from build123d import *

# Parameters (mm, degrees)
ESTRUSIONE_ESTRUSIONE1_DEPTH = 10
TAGLIO_ESTRUSIONE6_DEPTH     = 3.5
SCHIZZO3_R                   = 1.75
TAGLIO_ESTRUSIONE7_DEPTH     = 21.645708387
ESTRUSIONE_ESTRUSIONE2_DEPTH = 3
SCHIZZO5_R                   = 2
TAGLIO_ESTRUSIONE8_DEPTH     = 1.5
SMUSSO2_SIZE                 = 0.5
TAGLIO_ESTRUSIONE9_DEPTH     = 3.5


with BuildPart() as part:
    # Schizzo1 → Estrusione-Estrusione1 (new, symmetric)
    with BuildSketch(Plane.XY):
        Polygon((11, -1), (11, 0), (-11, 0), (-11, -1), (-15.041451884, -8), (-15.041451884, -10), (15.041451884, -10), (15.041451884, -8), align=None)
    extrude(amount=ESTRUSIONE_ESTRUSIONE1_DEPTH, both=True)

    # Schizzo2 → Taglio-Estrusione6 (cut, symmetric)
    with BuildSketch(Plane(origin=(0, 0, 0), x_dir=(0, 0, -1), z_dir=(1, 0, 0))):
        with BuildLine():
            Line((-10, 0), (-9.740175425, 0))
            ThreePointArc((-9.740175425, 0), (-9.641268354, -0.037228588), (-9.591456891, -0.130434783))
            ThreePointArc((-9.591456891, -0.130434783), (-9.557611714, -0.288062154), (-9.498876404, -0.438202247))
            ThreePointArc((-9.498876404, -0.438202247), (-9, -0.75), (-8.501123596, -0.438202247))
            ThreePointArc((-8.501123596, -0.438202247), (-8.442388286, -0.288062154), (-8.408543109, -0.130434783))
            ThreePointArc((-8.408543109, -0.130434783), (-8.358731646, -0.037228588), (-8.259824575, 0))
            Line((-8.259824575, 0), (-8, 0))
            Line((-8, 0), (-7.740175425, 0))
            ThreePointArc((-7.740175425, 0), (-7.641268354, -0.037228588), (-7.591456891, -0.130434783))
            ThreePointArc((-7.591456891, -0.130434783), (-7.557611714, -0.288062154), (-7.498876404, -0.438202247))
            ThreePointArc((-7.498876404, -0.438202247), (-7, -0.75), (-6.501123596, -0.438202247))
            ThreePointArc((-6.501123596, -0.438202247), (-6.442388286, -0.288062154), (-6.408543109, -0.130434783))
            ThreePointArc((-6.408543109, -0.130434783), (-6.358731646, -0.037228588), (-6.259824575, 0))
            Line((-6.259824575, 0), (-6, 0))
            Line((-6, 0), (-5.740175425, 0))
            ThreePointArc((-5.740175425, 0), (-5.641268354, -0.037228588), (-5.591456891, -0.130434783))
            ThreePointArc((-5.591456891, -0.130434783), (-5.557611714, -0.288062154), (-5.498876404, -0.438202247))
            ThreePointArc((-5.498876404, -0.438202247), (-5, -0.75), (-4.501123596, -0.438202247))
            ThreePointArc((-4.501123596, -0.438202247), (-4.442388286, -0.288062154), (-4.408543109, -0.130434783))
            ThreePointArc((-4.408543109, -0.130434783), (-4.358731646, -0.037228588), (-4.259824575, 0))
            Line((-4.259824575, 0), (-4, 0))
            Line((-4, 0), (-3.740175425, 0))
            ThreePointArc((-3.740175425, 0), (-3.641268354, -0.037228588), (-3.591456891, -0.130434783))
            ThreePointArc((-3.591456891, -0.130434783), (-3.557611714, -0.288062154), (-3.498876404, -0.438202247))
            ThreePointArc((-3.498876404, -0.438202247), (-3, -0.75), (-2.501123596, -0.438202247))
            ThreePointArc((-2.501123596, -0.438202247), (-2.442388286, -0.288062154), (-2.408543109, -0.130434783))
            ThreePointArc((-2.408543109, -0.130434783), (-2.358731646, -0.037228588), (-2.259824575, 0))
            Line((-2.259824575, 0), (-2, 0))
            Line((-2, 0), (-1.740175425, 0))
            ThreePointArc((-1.740175425, 0), (-1.641268354, -0.037228588), (-1.591456891, -0.130434783))
            ThreePointArc((-1.591456891, -0.130434783), (-1.557611714, -0.288062154), (-1.498876404, -0.438202247))
            ThreePointArc((-1.498876404, -0.438202247), (-1, -0.75), (-0.501123596, -0.438202247))
            ThreePointArc((-0.501123596, -0.438202247), (-0.442388286, -0.288062154), (-0.408543109, -0.130434783))
            ThreePointArc((-0.408543109, -0.130434783), (-0.358731646, -0.037228588), (-0.259824575, 0))
            Line((-0.259824575, 0), (0, 0))
            Line((0, 0), (0.259824575, 0))
            ThreePointArc((0.259824575, 0), (0.358731646, -0.037228588), (0.408543109, -0.130434783))
            ThreePointArc((0.408543109, -0.130434783), (0.442388286, -0.288062154), (0.501123596, -0.438202247))
            ThreePointArc((0.501123596, -0.438202247), (1, -0.75), (1.498876404, -0.438202247))
            ThreePointArc((1.498876404, -0.438202247), (1.557611714, -0.288062154), (1.591456891, -0.130434783))
            ThreePointArc((1.591456891, -0.130434783), (1.641268354, -0.037228588), (1.740175425, 0))
            Line((1.740175425, 0), (2, 0))
            Line((2, 0), (2.259824575, 0))
            ThreePointArc((2.259824575, 0), (2.358731646, -0.037228588), (2.408543109, -0.130434783))
            ThreePointArc((2.408543109, -0.130434783), (2.442388286, -0.288062154), (2.501123596, -0.438202247))
            ThreePointArc((2.501123596, -0.438202247), (3, -0.75), (3.498876404, -0.438202247))
            ThreePointArc((3.498876404, -0.438202247), (3.557611714, -0.288062154), (3.591456891, -0.130434783))
            ThreePointArc((3.591456891, -0.130434783), (3.641268354, -0.037228588), (3.740175425, 0))
            Line((3.740175425, 0), (4, 0))
            Line((4, 0), (4.259824575, 0))
            ThreePointArc((4.259824575, 0), (4.358731646, -0.037228588), (4.408543109, -0.130434783))
            ThreePointArc((4.408543109, -0.130434783), (4.442388286, -0.288062154), (4.501123596, -0.438202247))
            ThreePointArc((4.501123596, -0.438202247), (5, -0.75), (5.498876404, -0.438202247))
            ThreePointArc((5.498876404, -0.438202247), (5.557611714, -0.288062154), (5.591456891, -0.130434783))
            ThreePointArc((5.591456891, -0.130434783), (5.641268354, -0.037228588), (5.740175425, 0))
            Line((5.740175425, 0), (6, 0))
            Line((6, 0), (6.259824575, 0))
            ThreePointArc((6.259824575, 0), (6.358731646, -0.037228588), (6.408543109, -0.130434783))
            ThreePointArc((6.408543109, -0.130434783), (6.442388286, -0.288062154), (6.501123596, -0.438202247))
            ThreePointArc((6.501123596, -0.438202247), (7, -0.75), (7.498876404, -0.438202247))
            ThreePointArc((7.498876404, -0.438202247), (7.557611714, -0.288062154), (7.591456891, -0.130434783))
            ThreePointArc((7.591456891, -0.130434783), (7.641268354, -0.037228588), (7.740175425, 0))
            Line((7.740175425, 0), (8, 0))
            Line((8, 0), (8.259824575, 0))
            ThreePointArc((8.259824575, 0), (8.358731646, -0.037228588), (8.408543109, -0.130434783))
            ThreePointArc((8.408543109, -0.130434783), (8.442388286, -0.288062154), (8.501123596, -0.438202247))
            ThreePointArc((8.501123596, -0.438202247), (9, -0.75), (9.498876404, -0.438202247))
            ThreePointArc((9.498876404, -0.438202247), (9.557611714, -0.288062154), (9.591456891, -0.130434783))
            ThreePointArc((9.591456891, -0.130434783), (9.641268354, -0.037228588), (9.740175425, 0))
            Line((9.740175425, 0), (10, 0))
            Line((10, 0), (10, 1.47712545))
            Line((10, 1.47712545), (-10, 1.47712545))
            Line((-10, 1.47712545), (-10, 0))
        make_face()
    extrude(amount=TAGLIO_ESTRUSIONE6_DEPTH, both=True, mode=Mode.SUBTRACT)

    # Schizzo3 → Taglio-Estrusione7 (cut, through all)
    with BuildSketch(Plane(origin=(0, 0, 0), x_dir=(1, 0, 0), z_dir=(0, 1, 0))):
        with Locations(Location((7.25, 6.25, 0), (0, 0, 180))):
            Circle(SCHIZZO3_R)
        with Locations(Location((7.25, -6.25, 0), (0, 0, 180))):
            Circle(SCHIZZO3_R)
        with Locations(Location((-7.25, -6.25, 0), (0, 0, 180))):
            Circle(SCHIZZO3_R)
        with Locations(Location((-7.25, 6.25, 0), (0, 0, 180))):
            Circle(SCHIZZO3_R)
    extrude(amount=-TAGLIO_ESTRUSIONE7_DEPTH, mode=Mode.SUBTRACT)

    # Schizzo4 → Estrusione-Estrusione2 (add)
    with BuildSketch(Plane.XY.offset(10)):
        Polygon((-15.041451884, -10), (15.041451884, -10), (15.041451884, -8), (11, -1), (11, 3), (3.994785695, 3), (3.994785695, -1), (-4.005214305, -1), (-4.005214305, 3), (-11, 3), (-11, -1), (-15.041451884, -8), align=None)
    extrude(amount=ESTRUSIONE_ESTRUSIONE2_DEPTH)

    # Schizzo5 → Taglio-Estrusione8 (cut)
    with BuildSketch(Plane.XY.offset(13)):
        with Locations((7.497392847, -1)):
            Circle(SCHIZZO5_R)
        with Locations((-7.502607153, -1)):
            Circle(SCHIZZO5_R)
    extrude(amount=-TAGLIO_ESTRUSIONE8_DEPTH, mode=Mode.SUBTRACT)

    # Smusso2
    smusso2_edges = [part.edges().sort_by_distance(p)[0] for p in [
        (5.497392847, -1, 13),
        (-9.502607153, -1, 13),
    ]]
    chamfer(smusso2_edges, length=SMUSSO2_SIZE)

    # Schizzo6 → Taglio-Estrusione9 (cut)
    with BuildSketch(Plane.XZ.offset(10)):
        Polygon((-8.9, 9.107883832), (-10.55, 6.25), (-8.9, 3.392116168), (-5.6, 3.392116168), (-3.95, 6.25), (-5.6, 9.107883832), align=None)
        Polygon((-5.6, -3.392116168), (-8.9, -3.392116168), (-10.55, -6.25), (-8.9, -9.107883832), (-5.6, -9.107883832), (-3.95, -6.25), align=None)
        Polygon((10.55, -6.25), (8.9, -3.392116168), (5.6, -3.392116168), (3.95, -6.25), (5.6, -9.107883832), (8.9, -9.107883832), align=None)
        Polygon((5.6, 3.392116168), (8.9, 3.392116168), (10.55, 6.25), (8.9, 9.107883832), (5.6, 9.107883832), (3.95, 6.25), align=None)
    extrude(amount=-TAGLIO_ESTRUSIONE9_DEPTH, mode=Mode.SUBTRACT)


solid = part.part
The model under review builds one solid part; all positions refer to its coordinate system, in mm. A direction names the side the tool comes from. Round coordinates to 2 decimals unless told otherwise and drop trailing zeros. Loops run counter-clockwise (first coordinate to the right, second up) from the corner with the lowest first, then second, coordinate; pieces in that order, holes last. Notation, with made-up numbers: (33.25, -11.75) -> (79.25, -11.75) arc R16 cw to (79.25, 0.25) -> close; hole circle Ø2 at (22, -2.75). An arc over 180 degrees is marked (long way). Write item = value, one per line. Start each with the question number.
Item 1: Take a section at C-C on x = 8. Count the separate pieces of the cut face and the enclosed holes in it, plus the area to 3 significant figures.
Item 2: For faces 4 (the flat face through (-4.787, -8.274, 4.801)), 5 (the cylindrical face through (0.05, -0.75, -0.99)), 6 (the cylindrical face through (-8.06, -3.2, 4.7)), list the 3-axis set-ups (+Z, -Z, +X, -X, +Y, -Y) from which the entire face can be reached by the end or side of a thin tool; tool diameter is ignored.
Item 3: Take a section at B-B on z = 11. Give the boundary of the cut face in (x, y).
Item 4: Mouldability with a two-part tool opening along X and no side actions: class faces 1 (the flat face through (-4.787, -8.274, -7.699)), 2 (the flat face through (0, -5, 13)), 3 (the flat face through (-12.99, -4.45, 1.34)) as released by +X, released by -X, zero draft, split by the parting line, or undercut.
Item 5: Insertion check: pin 1 (5 mm diameter, centred on y = -2, z = 3.5, fed in from -X); pin 2 (0.8 mm diameter, centred on y = -0.5, z = 1, fed in from +X); pin 3 (10 mm diameter, centred on x = -2.5, z = -1, fed in from +Y). Each pin has a flat end and moves straight along its axis. Give the tip position at first contact, or say it passes through.
Item 6: Take a section at A-A on y = -5. Give the boundary of the cut face in (x, z), plus the area to 3 significant figures.
Item 7: To check wall thickness, follow L1, parallel to X at y = -0.5, z = -2.75; L2, parallel to Z at x = -6, y = -6.25; L3, parallel to X at y = -6.25, z = -5.5. State the ranges of each line that lie inside material, in increasing order.
Item 8: Take a section at D-D on x = 13.5. Give the boundary of the cut face in (y, z).
Result:
q1.separate_pieces = 3
q1.enclosed_holes = 0
q1.area = 152 mm²
q2.face_4 = -Y
q2.face_5 = +Y
q2.face_6 = +Y, -Y
q3.outline = (-15.04, -10) -> (15.04, -10) -> (15.04, -8) -> (11, -1) -> (11, 3) -> (3.99, 3) -> (3.99, -1) -> (-4.01, -1) -> (-4.01, 3) -> (-11, 3) -> (-11, -1) -> (-15.04, -8) -> close
q4.face_1 = undercut
q4.face_2 = zero draft
q4.face_3 = released by -X
q5.pin_1 = -13.02
q5.pin_2 = 11
q5.pin_3 = 0
q6.outline = (-13.31, -10) -> (13.31, -10) -> (13.31, 13) -> (-13.31, 13) -> close; hole circle Ø3.5 at (-7.25, -6.25); hole circle Ø3.5 at (-7.25, 6.25); hole circle Ø3.5 at (7.25, -6.25); hole circle Ø3.5 at (7.25, 6.25)
q6.area = 574 mm²
q7.L1 = -11 to -3.5, 3.5 to 11
q7.L2 = -10 to -7.47, -5.03 to 5.03, 7.47 to 13
q7.L3 = -14.03 to -8.83, -5.67 to 5.67, 8.83 to 14.03
q8.outline = (-10, -10) -> (-5.33, -10) -> (-5.33, 13) -> (-10, 13) -> close
